Autodesk Inventor part; units mm, degrees
ref_plane "YZ Plane" through (0, 0, 0) normal (1, 0, 0) x (0, 1, 0)
ref_plane "XZ Plane" through (0, 0, 0) normal (0, 1, 0) x (-1, 0, 0)
ref_plane "XY Plane" through (0, 0, 0) normal (0, 0, 1) x (1, 0, 0)
sketch "Sketch1" plane through (0, 0, 0) normal (0, 1, 0) x (-1, 0, 0)
  line L0 (15, 32.5) -> (-15, 32.5)
  line L1 (-15, 32.5) -> (-15, -32.5)
  line L2 (-15, -32.5) -> (15, -32.5)
  line L3 (15, -32.5) -> (15, 32.5)
  point P0 (0, 0)
  dimension "d0" = 65
  dimension "d1" = 30
  dimension "d2" = 15
  dimension "d3" = 32.5
extrude "Extrusion1" add sketch "Sketch1" along normal blind 12.7
sketch "Sketch2" plane through (0, 0, 0) normal (0, -1, 0) x (1, 0, 0)
  line L0 (8.07, 8.904) -> (-4.13, 8.904)
  line L1 (-4.13, 8.904) -> (-4.13, -3.296)
  line L2 (-4.13, -3.296) -> (8.07, -3.296)
  line L3 (8.07, -3.296) -> (8.07, 8.904)
  line L4 (-15, 32.5) -> (15, 32.5)
  line L5 (15, 32.5) -> (15, -32.5)
  point P0 (0, 0)
  dimension "d6" = 12.2
  dimension "d7" = 12.2
  dimension "d8" = 23.596
  dimension "d9" = 6.93
extrude "Extrusion2" add sketch "Sketch2" along normal blind 0.716
sketch "Sketch3" plane through (0, 0, 0) normal (0, -1, 0) x (1, 0, 0)
  line L0 (15, 32.5) -> (15, -32.5)
  line L1 (15, 25.85) -> (7.4, 25.85)
  line L2 (7.4, 25.85) -> (7.4, 14.15)
  line L3 (7.4, 14.15) -> (15, 14.15)
  line L4 (15, 14.15) -> (15, 25.85)
  line L5 (-15, 32.5) -> (15, 32.5)
  point P0 (0, 0)
  dimension "d12" = 7.6
  dimension "d13" = 11.7
  dimension "d14" = 6.65
extrude "Extrusion3" cut sketch "Sketch3" against normal blind 5
sketch "Sketch4" plane through (0, 0, 0) normal (0, -1, 0) x (1, 0, 0)
  line L0 (15, 14.15) -> (15, -32.5)
  line L1 (15, -4.75) -> (10.3, -4.75)
  line L2 (10.3, -4.75) -> (10.3, -13.05)
  line L3 (10.3, -13.05) -> (15, -13.05)
  line L4 (15, -13.05) -> (15, -4.75)
  line L5 (-15, 32.5) -> (15, 32.5)
  point P0 (0, 0)
  dimension "d17" = 4.7
  dimension "d18" = 8.3
  dimension "d19" = 37.25
extrude "Extrusion4" cut sketch "Sketch4" against normal blind 4.3
sketch "Sketch5" plane through (0, 0, 0) normal (0, -1, 0) x (1, 0, 0)
  line L0 (15, -13.05) -> (15, -32.5)
  line L1 (15, -17.35) -> (10.3, -17.35)
  line L2 (10.3, -17.35) -> (10.3, -25.65)
  line L3 (10.3, -25.65) -> (15, -25.65)
  line L4 (15, -25.65) -> (15, -17.35)
  line L5 (15, -32.5) -> (-15, -32.5)
  point P0 (0, 0)
  dimension "d22" = 4.7
  dimension "d23" = 8.3
  dimension "d24" = 6.85
extrude "Extrusion5" cut sketch "Sketch5" against normal blind 4.3
sketch "Sketch6" plane through (0, 0, 0) normal (0, -1, 0) x (1, 0, 0)
  circle A0 centre (11.5, 29) radius 3
  circle A1 centre (-11.5, 29) radius 3
  circle A2 centre (-11.5, -29) radius 3
  circle A3 centre (11.5, -29) radius 3
  line L0 (15, -32.5) -> (-15, -32.5)
  line L1 (-15, -32.5) -> (-15, 32.5)
  line L2 (-15, 32.5) -> (15, 32.5)
  point P0 (0, 0)
  dimension "d27" = 6
  dimension "d28" = 6
  dimension "d29" = 6
  dimension "d30" = 6
  dimension "d31" = 0
  dimension "d32" = 23
  dimension "d33" = 58
  dimension "d34" = 3.5
  dimension "d35" = 23
  dimension "d37" = 0
  dimension "d38" = 3.5
  dimension "d42" = 3.5
extrude "Extrusion6" add sketch "Sketch6" along normal blind 4.595
sketch "Sketch7" plane through (11.5, -4.595, 29) normal (0, -1, 0) x (1, 0, 0)
  circle A0 centre (0, 0) radius 3
  circle A1 centre (0, -58) radius 3
  circle A2 centre (-23, -58) radius 3
  circle A3 centre (-23, 0) radius 3
  point P0 (-11.5, -29)
hole "Hole1" at (11.5, -4.595, 29) at (-11.5, -4.595, 29) at (-11.5, -4.595, -29) at (11.5, -4.595, -29) direction (0, 1, 0) diameter 2.75 depth 25.4 tip angle 118
sketch "Sketch8" plane through (0, 0, 0) normal (0, -1, 0) x (1, 0, 0)
  line L0 (15, -32.5) -> (-15, -32.5)
  line L1 (8.255, -32.5) -> (-8.255, -32.5)
  line L2 (-8.255, -32.5) -> (-8.255, -27.166)
  line L3 (-8.255, -27.166) -> (8.255, -27.166)
  line L4 (8.255, -27.166) -> (8.255, -32.5)
  point P0 (0, 0)
  point P1 (0, 0)
  dimension "d50" = 5.334
  dimension "d51" = 16.51
  dimension "d52" = 8.255
extrude "Extrusion7" cut sketch "Sketch8" against normal blind 2.032
sketch "Sketch9" plane through (0, 0, 0) normal (0, -1, 0) x (1, 0, 0)
  line L0 (4.228, 30.9) -> (-7.722, 30.9)
  line L1 (-7.722, 30.9) -> (-7.722, 19.5)
  line L2 (-7.722, 19.5) -> (4.228, 19.5)
  line L3 (4.228, 19.5) -> (4.228, 30.9)
  line L4 (-15, 32.5) -> (15, 32.5)
  line L5 (-15, -32.5) -> (-15, 32.5)
  line L6 (15, 32.5) -> (15, 25.85)
  point P0 (0, 0)
  dimension "d56" = 1.6
  dimension "d57" = 11.4
  dimension "d58" = 11.95
  dimension "d60" = 10.772
extrude "Extrusion8" add sketch "Sketch9" along normal blind 3.175
equation "\"d6\" = d7"
equation "\"d28\" = d27"
equation "\"d29\" = d27"
equation "\"d30\" = d27"
equation "\"d35\" = d32"
properties part number "Heat Block for Pi" material "Aluminum 6061"
Here's how the part is built. I have some questions about the finished solid (model axes, mm). A direction names the side the tool comes from. Give positions to 0.01 mm unless a question says otherwise; leave off trailing zeros. Write each loop counter-clockwise with the first axis right and the second up, starting at its lowest first coordinate (ties: lowest second). Pieces come first, ordered by that corner, then holes. Notation, with made-up numbers: (-29, 44.25) -> (16, 44.25) arc R23 cw to (16, 52.25) -> close; hole circle Ø1 at (-4.5, -18). An arc over 180 degrees is marked (long way). Use one line per item in the form item = value. Start each with the question number.
1. If I drill on L1, parallel to X at y = 5, z = -29 (3 decimals); L2, parallel to Z at x = -11.5, y = 2.5 (3 decimals); L3, parallel to X at y = 0.25, z = -29 (3 decimals), over which ranges is the centre line in solid material (lowest first)?
2. Imagine slicing it at D-D on z = -18. List the corners of the cut face in (x, y) for me, plus the area to 3 significant figures.
3. Thinking about a two-plate mould opening in X: for faces 1 (the face through (11, 2, 25.85)), 2 (the face through (10.3, 2, -9)), 3 (the face through (-11.56, 4.174, -27.626)), which applies, +X half, -X half, draft (parallel to the pull), parting line (faces both ways), or undercut?
4. Imagine slicing it at B-B on y = 3. List the corners of the cut face in (x, z) for me (3 decimals).
5. On a 3-axis mill with a long thin cutter (end or side, diameter ignored), from which of +Z, -Z, +X, -X, +Y, -Y can I reach the whole of each face in a straight line? I mean faces 4 (the face through (13, 4.3, -21)), 5 (the face through (-13.9, -2.3, -27.2)), 6 (the face through (-2, -3.175, 25)), 7 (the face through (4.228, -2, 25)), 8 (the face through (0, 2.032, -30)). Say none if no direction works.
6. Imagine slicing it at A-A on z = 29. List the corners of the cut face in (x, y) for me (3 decimals).
7. Imagine slicing it at C-C on x = 11.5. State how many separate pieces and enclosed holes the cut face has, plus the area to 3 significant figures.
8. Will these pins go through, and if not, where does the flat tip stop? pin 1 Ø2.5 at (y, z) = (-2.5, 27.5) entering from +X; pin 2 Ø9 at (x, z) = (-1, 26.5) entering from -Y (3 decimals); pin 3 Ø2.5 at (x, y) = (-4, -1.5) entering from -Z.
Entries:
q1.L1 = -15 to -12.875, -10.125 to 10.125, 12.875 to 15
q1.L2 = -32.5 to -30.375, -27.625 to 27.625, 30.375 to 32.5
q1.L3 = -15 to -12.875, -10.125 to -8.255, 8.255 to 10.125, 12.875 to 15
q2.outline = (-15, 0) -> (10.3, 0) -> (10.3, 4.3) -> (15, 4.3) -> (15, 12.7) -> (-15, 12.7) -> close
q2.area = 361 mm²
q3.face_1 = draft
q3.face_2 = +X half
q3.face_3 = undercut
q4.outline = (-15, -32.5) -> (15, -32.5) -> (15, -25.65) -> (10.3, -25.65) -> (10.3, -17.35) -> (15, -17.35) -> (15, -13.05) -> (10.3, -13.05) -> (10.3, -4.75) -> (15, -4.75) -> (15, 14.15) -> (7.4, 14.15) -> (7.4, 25.85) -> (15, 25.85) -> (15, 32.5) -> (-15, 32.5) -> close; hole circle Ø2.75 at (-11.5, -29); hole circle Ø2.75 at (-11.5, 29); hole circle Ø2.75 at (11.5, -29); hole circle Ø2.75 at (11.5, 29)
q5.face_4 = +X, -Y
q5.face_5 = -Y
q5.face_6 = +Z, -Z, -Y
q5.face_7 = +Z, -Y
q5.face_8 = -Z, -Y
q6.outline = (-15, 0) -> (-14.5, 0) -> (-14.5, -4.595) -> (-12.875, -4.595) -> (-12.875, 12.7) -> (-15, 12.7) -> close; (-10.125, -4.595) -> (-8.5, -4.595) -> (-8.5, 0) -> (-7.722, 0) -> (-7.722, -3.175) -> (4.228, -3.175) -> (4.228, 0) -> (8.5, 0) -> (8.5, -4.595) -> (10.125, -4.595) -> (10.125, 12.7) -> (-10.125, 12.7) -> close; (12.875, -4.595) -> (14.5, -4.595) -> (14.5, 0) -> (15, 0) -> (15, 12.7) -> (12.875, 12.7) -> close
q7.separate_pieces = 3
q7.enclosed_holes = 0
q7.area = 656 mm²
q8.pin_1 = 14.49
q8.pin_2 = -3.175
q8.pin_3 = -3.3
